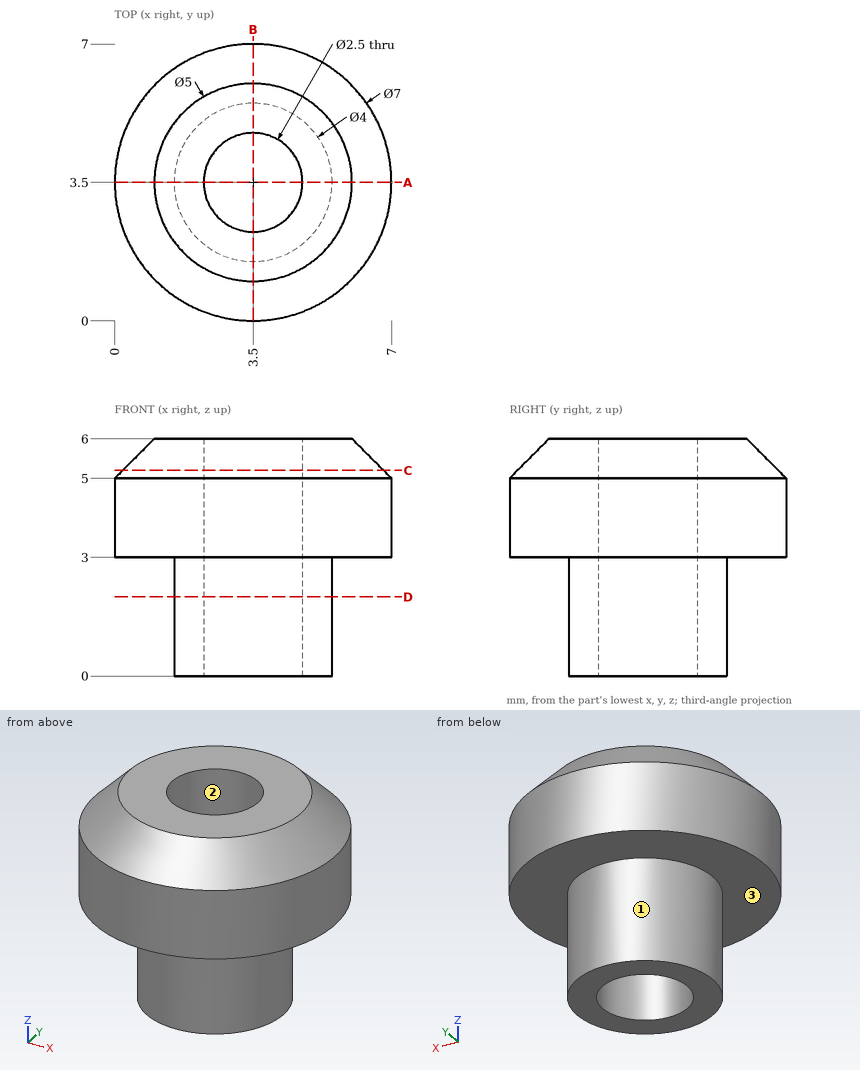
Source: three-view drawing plus pictorial views. Frame: mm from the lowest corner of the part. Give positions to 0.01 mm unless a question says otherwise; leave off trailing zeros. Order: outer loops, then holes, each group sorted by start corner. A loop starts at its lowest first (then second) coordinate and runs counter-clockwise, first axis right, second up.
1. Material intervals for L1, parallel to Y at x = 3.5, z = 2.8; L2, parallel to Z at x = 3, y = 5.75; L3, parallel to X at y = 4, z = 5.3, sorted ascending.
Derived:
L1: y = 1.5 to 2.25, 4.75 to 5.5
L2: z = 3 to 6
L3: x = 0.34 to 2.35, 4.65 to 6.66
2. Pin query (flat end, axial travel): pin 1 (3 mm diameter, centred on y = 5, z = 0.5, fed in from -X); pin 2 (1.5 mm diameter, centred on y = 1, z = 1.5, fed in from +X); pin 3 (2 mm diameter, centred on y = 2, z = 4.5, fed in from +X). Return the tip coordinate at first contact, or that it passes through.
Derived:
pin 1: stops at x = 1.5
pin 2: stops at x = 4.47
pin 3: stops at x = 6.96
3. Section C-C on z = 5.2. Return the cut outline in (x, y).
Derived:
outline: circle Ø6.6 at (3.5, 3.5); hole circle Ø2.5 at (3.5, 3.5)
4. Section D-D on z = 2. Return the cut outline in (x, y).
Derived:
outline: circle Ø4 at (3.5, 3.5); hole circle Ø2.5 at (3.5, 3.5)
5. Mould query, pull axis X, two halves, no side actions, for the marked faces 1, 2 and 3. Classes: released by +X, released by -X, zero draft, split by the parting line, or undercut.
Derived:
face 1: split by the parting line
face 2: undercut
face 3: zero draft
6. Section A-A on y = 3.5. Return the cut outline in (x, z), and give its area (3 significant figures).
Derived:
outline: (0, 3) - (1.5, 3) - (1.5, 0) - (2.25, 0) - (2.25, 6) - (1, 6) - (0, 5) - close; (4.75, 0) - (5.5, 0) - (5.5, 3) - (7, 3) - (7, 5) - (6, 6) - (4.75, 6) - close
area: 17.0 mm2
